```python
from build123d import *

# Parameters (mm, degrees)
SALIENTE_EXTRUIR1_DEPTH = 14.5
CROQUIS3_R              = 30
CORTAR_EXTRUIR1_DEPTH   = 59.39734583
CROQUIS4_R              = 1.35
CORTAR_EXTRUIR2_DEPTH   = 30


with BuildPart() as part:
    # Croquis1 → Saliente-Extruir1 (new body)
    with BuildSketch(Plane(origin=(0, 0, 0), x_dir=(1, 0, 0), z_dir=(0, 1, 0))):
        with BuildLine():
            Line((-40, 0), (-40, 40))
            Line((-40, 40), (40, 40))
            Line((40, 40), (40, 0))
            ThreePointArc((40, 0), (0, -40), (-40, 0))
        make_face()
    extrude(amount=SALIENTE_EXTRUIR1_DEPTH)

    # Croquis3 → Cortar-Extruir1 (cut, through all)
    with BuildSketch(Plane(origin=(0, 14.5, 0), x_dir=(1, 0, 0), z_dir=(0, 1, 0))):
        with Locations(Location((0, 0, 0), (0, 0, 270))):
            Circle(CROQUIS3_R)
    extrude(amount=-CORTAR_EXTRUIR1_DEPTH, mode=Mode.SUBTRACT)

    # Croquis4 → Cortar-Extruir2 (cut)
    with BuildSketch(Plane(origin=(0, 0, -40), x_dir=(-1, 0, 0), z_dir=(0, 0, -1))):
        with Locations((-35, 9.5)):
            Circle(CROQUIS4_R)
        with Locations((-35, 5)):
            Circle(CROQUIS4_R)
        with Locations((35, 9.5)):
            Circle(CROQUIS4_R)
        with Locations((35, 5)):
            Circle(CROQUIS4_R)
    extrude(amount=-CORTAR_EXTRUIR2_DEPTH, mode=Mode.SUBTRACT)


solid = part.part
```
CAD build for the part. Positions are in the model's coordinates, mm. A direction names the side the tool comes from. Coordinates: 2 decimals unless noted, no trailing zeros. Order: outer loops, then holes, each group sorted by start corner. A loop starts at its lowest first (then second) coordinate and runs counter-clockwise, first axis right, second up. Notation, with made-up numbers: (14.5, 14.5) -> (66.5, 14.5) arc R18 ccw to (66.5, 21.5) -> close; hole circle Ø1 at (-40, -36.5). An arc over 180 degrees is marked (long way). Use one line per item in the form item = value. Start each with the question number.
1) Band-saw the part on B-B on x = 0. Give the cut face in (y, z).
2) Drill centre lines: L1, parallel to Y at x = 35, z = -32.25; L2, parallel to X at y = 10.5, z = -11; L3, parallel to X at y = 8.5, z = -0.5. Where is each one in solid material? Low to high. Write a range as [from, to].
3) Band-saw the part on C-C on y = 9.5. Give the cut face in (x, z).
4) Band-saw the part on D-D on z = 22. Give the cut face in (x, y), then the cut area to 3 significant figures.
5) Tool access for faces 1 (the cylindrical face through (1.32, 7.35, -29.97)), 2 (the cylindrical face through (34.274, 6.138, -25.21)): list every direction of +Z, -Z, +X, -X, +Y, -Y with a clear straight run to the whole face (end or side of a thin tool).
6) Drop flat-ended pins along their axis: pin 1 (1.5 mm diameter, centred on y = 4, z = 1, fed in from -X); pin 2 (2.5 mm diameter, centred on x = 35, y = 5, fed in from +Z); pin 3 (3.5 mm diameter, centred on x = 35, y = 9.5, fed in from +Z). Give the stop position or say it passes through.
7) Pull direction Y, two halves, no side cores. Call faces 3 (the flat face through (-35, 5, -10)), 4 (the flat face through (-1, 7, -40)), 5 (the flat face through (-17, 0, -27)): +Y half, -Y half, draft (parallel to the pull), parting line (faces both ways), or undercut.
8) Band-saw the part on A-A on z = -18. Give the cut face in (x, y), then the cut area to 3 significant figures.
Entries:
q1.outline = (0, -40) -> (14.5, -40) -> (14.5, -30) -> (0, -30) -> close; (0, 30) -> (14.5, 30) -> (14.5, 40) -> (0, 40) -> close
q2.L1 = [0, 3.65], [6.35, 8.15], [10.85, 14.5]
q2.L2 = [-40, -35.91], [-34.09, -27.91], [27.91, 34.09], [35.91, 40]
q2.L3 = [-40, -30], [30, 40]
q3.outline = (-40, -40) -> (-36.35, -40) -> (-36.35, -10) -> (-33.65, -10) -> (-33.65, -40) -> (33.65, -40) -> (33.65, -10) -> (36.35, -10) -> (36.35, -40) -> (40, -40) -> (40, 0) arc R40 ccw to (-40, 0) -> close; hole circle Ø60 at (0, 0)
q4.outline = (-33.41, 0) -> (-20.4, 0) -> (-20.4, 14.5) -> (-33.41, 14.5) -> close; (20.4, 0) -> (33.41, 0) -> (33.41, 14.5) -> (20.4, 14.5) -> close
q4.area = 377 mm2
q5.face_1 = +Y, -Y
q5.face_2 = -Z
q6.pin_1 = -40
q6.pin_2 = 21.47
q6.pin_3 = 22.24
q7.face_3 = undercut
q7.face_4 = draft
q7.face_5 = -Y half
q8.outline = (-40, 0) -> (-24, 0) -> (-24, 14.5) -> (-40, 14.5) -> close; (24, 0) -> (40, 0) -> (40, 14.5) -> (24, 14.5) -> close; hole circle Ø2.7 at (-35, 5); hole circle Ø2.7 at (-35, 9.5); hole circle Ø2.7 at (35, 5); hole circle Ø2.7 at (35, 9.5)
q8.area = 441 mm2
